The model under review builds one solid part; all positions refer to its coordinate system, in mm. A direction names the side the tool comes from. Round coordinates to 2 decimals unless told otherwise and drop trailing zeros. Order: outer loops, then holes, each group sorted by start corner. A loop starts at its lowest first (then second) coordinate and runs counter-clockwise, first axis right, second up. Notation, with made-up numbers: M 17.5,11.5 L 62.5,11.5 A29 cw 62.5,36.5 Z; hole C -33.75,-12.75 d8. An arc over 180 degrees is marked long. Use a Markdown table: item, result. Add a question column.
1. Insertion check: P1, Ø3, axis at y = -5, z = 5, coming from the -X side; P2, Ø6, axis at x = -8.5, z = 24, coming from the -Y side; P3, Ø1, axis at y = 7, z = 27, coming from the +X side; P4, Ø4, axis at x = 18.575, z = 22.5, coming from the -Y side. Each pin has a flat end and moves straight along its axis. Give the tip position at first contact, or say it passes through.
2. The part is to be moulded in two halves that separate along Z. For faces 3 (the flat face through (0, 6, 30)), 4 (the cylindrical face through (13.83, 1.2, 22.67)), 5 (the flat face through (-19, -8.55, 15)), say which applies: +Z half, -Z half, draft (parallel to the pull), parting line (faces both ways), or undercut.
3. To check wall thickness, follow probe 1 along Z at (x, y) = (-20.5, -7.75); probe 2 along X at (y, z) = (-6, 7.5) (3 decimals); probe 3 along X at (y, z) = (-4.5, 22.5) (3 decimals). State the ranges of each line that lie inside material, in increasing order.
4. Consider section C-C on y = 3. State the section outline as (x, z) points (3 decimals).
5. Consider section A-A on y = -3.75. State the section outline as (x, z) points (3 decimals), then the cut area to 3 significant figures.
6. For faces 1 (the flat face through (21, -2.25, 24)), 2 (the flat face through (-18.04, 2.71, 14.94)), list the 3-axis set-ups (+Z, -Z, +X, -X, +Y, -Y) from which the entire face can be reached by the end or side of a thin tool; tool diameter is ignored.
7. Consider section B-B on z = 22.5. State the section outline as (x, y) points (3 decimals).
from build123d import *

# Parameters (mm, degrees)
SKETCH1_W              = 48
SKETCH1_H              = 17.5
BODY_DEPTH             = 30
TUBE_CUTOUT_DEPTH      = 40.402569713
SKETCH3_R              = 2.65
CUT_EXTRUDE_M5_DEPTH   = 43.216702856
SLOPE_DEPTH            = 40.402569713
BOLT_HEAD_CUTOUT_START = -6.5
SKETCH5_R              = 4.75
BOLT_HEAD_CUTOUT_DEPTH = 23
FILLET_2_R             = 10
SKETCH7_W              = 48
SKETCH7_H              = 30
CLEARANCE_DEPTH        = 0.2


with BuildPart() as part:
    # Sketch1 → body (new body)
    with BuildSketch(Plane.XY):
        Rectangle(SKETCH1_W, SKETCH1_H)
    extrude(amount=BODY_DEPTH)

    # Sketch2 → tube_cutout (cut, through all)
    with BuildSketch(Plane.XY):
        with BuildLine():
            Line((13.15, -8.75), (-13.15, -8.75))
            ThreePointArc((-13.15, -8.75), (0, 4.4), (13.15, -8.75))
        make_face()
    extrude(amount=TUBE_CUTOUT_DEPTH, mode=Mode.SUBTRACT)

    # Sketch3 → Cut-Extrude M5 (cut, through all)
    with BuildSketch(Plane.XZ.offset(8.75)):
        with Locations(Location((18.575, 22.5, 0), (0, 0, 270))):
            Circle(SKETCH3_R)
        with Locations(Location((18.575, 7.5, 0), (0, 0, 270))):
            Circle(SKETCH3_R)
        with Locations(Location((-18.575, 7.5, 0), (0, 0, 90))):
            Circle(SKETCH3_R)
        with Locations(Location((-18.575, 22.5, 0), (0, 0, 90))):
            Circle(SKETCH3_R)
    extrude(amount=-CUT_EXTRUDE_M5_DEPTH, mode=Mode.SUBTRACT)

    # Sketch4 → slope (cut, through all)
    with BuildSketch(Plane.XY):
        Polygon((-24, 8.75), (-24, -3.25), (-12, 8.75), align=None)
        Polygon((24, -3.25), (12, 8.75), (24, 8.75), align=None)
    extrude(amount=SLOPE_DEPTH, mode=Mode.SUBTRACT)

    # Sketch5 → bolt_head_cutout (cut)
    with BuildSketch(Plane.XZ.offset(8.75).offset(BOLT_HEAD_CUTOUT_START)):
        with Locations((18.575, 22.5)):
            Circle(SKETCH5_R)
        with Locations((18.575, 7.5)):
            Circle(SKETCH5_R)
        with Locations((-18.575, 7.5)):
            Circle(SKETCH5_R)
        with Locations((-18.575, 22.5)):
            Circle(SKETCH5_R)
    extrude(amount=-BOLT_HEAD_CUTOUT_DEPTH, mode=Mode.SUBTRACT)

    # fillet 2
    # the kernel refuses this fillet: 10 mm, written as the material it takes off along each edge
    with BuildSketch(Plane(origin=(24, -3.25, -10.355339059), x_dir=(-0.7071067811865475, 0.7071067811865478, 0), z_dir=(0, 0, 1)), Plane(origin=(12, 8.75, -10.355339059), x_dir=(-1, 0, 0), z_dir=(0, 0, 1)), Plane(origin=(-12, 8.75, -10.355339059), x_dir=(-0.7071067811865474, -0.7071067811865478, 0), z_dir=(0, 0, 1))) as fillet_2_piece_1:
        with BuildLine():
            CenterArc((FILLET_2_R * 0.414213562373, FILLET_2_R), FILLET_2_R, 225, 45)
            Line((-FILLET_2_R * 0.292893218813, FILLET_2_R * 0.292893218813), (0, 0))
            Line((0, 0), (FILLET_2_R * 0.414213562373, 0))
        make_face()
    extrude(amount=50.710678119, mode=Mode.SUBTRACT)
    with BuildSketch(Plane(origin=(-24, -3.25, -10.355339059), x_dir=(0.7071067811865469, 0.707106781186548, 0), z_dir=(0, 0, 1))) as fillet_2_piece_2:
        with BuildLine():
            CenterArc((FILLET_2_R * 0.414213562373, -FILLET_2_R), FILLET_2_R, 90, 45)
            Line((-FILLET_2_R * 0.292893218813, -FILLET_2_R * 0.292893218813), (0, 0))
            Line((0, 0), (FILLET_2_R * 0.414213562373, 0))
        make_face()
    extrude(amount=50.710678119, mode=Mode.SUBTRACT)

    # Sketch7 → clearance (cut)
    with BuildSketch(Plane.XZ.offset(8.75)):
        with Locations((0, 15)):
            Rectangle(SKETCH7_W, SKETCH7_H)
    extrude(amount=-CLEARANCE_DEPTH, mode=Mode.SUBTRACT)


solid = part.part
Answer block:
| question | item | result |
|---|---|---|
| 1 | P1 | x = -23.96 |
| 1 | P2 | y = -2.37 |
| 1 | P3 | x = 14.18 |
| 1 | P4 | through |
| 2 | face 3 | +Z half |
| 2 | face 4 | undercut |
| 2 | face 5 | draft |
| 3 | probe 1 | 0 to 5.68, 9.32 to 20.68, 24.32 to 30 |
| 3 | probe 2 | -23.903 to -21.225, -15.925 to -12.859, 12.859 to 15.925, 21.225 to 23.903 |
| 3 | probe 3 | -23.573 to -21.225, -15.925 to -12.444, 12.444 to 15.925, 21.225 to 23.573 |
| 4 | outline | M -17.75,0 L -5.904,0 L -5.904,30 L -17.75,30 L -17.75,27.178 A4.75 cw -17.75,17.822 L -17.75,12.178 A4.75 cw -17.75,2.822 Z; M 5.904,0 L 17.75,0 L 17.75,2.822 A4.75 cw 17.75,12.178 L 17.75,17.822 A4.75 cw 17.75,27.178 L 17.75,30 L 5.904,30 Z |
| 5 | outline | M -23.313,0 L -12.162,0 L -12.162,30 L -23.313,30 Z; M 12.162,0 L 23.313,0 L 23.313,30 L 12.162,30 Z; hole C -18.575,7.5 d5.3; hole C -18.575,22.5 d5.3; hole C 18.575,7.5 d5.3; hole C 18.575,22.5 d5.3 |
| 5 | area | 581 mm^2 |
| 6 | face 1 | +Y |
| 6 | face 2 | +Z, -Z, -X, +Y |
| 7 | outline | M -24,-8.55 L -21.225,-8.55 L -21.225,-2.25 L -22.577,-2.25 A10 ccw -24,-7.392 Z; M -15.925,-8.55 L -13.148,-8.55 A13.15 cw 13.148,-8.55 L 15.925,-8.55 L 15.925,-2.25 L 13.825,-2.25 L 13.825,6.775 A10 ccw 7.858,8.75 L -7.858,8.75 A10 ccw -13.825,6.775 L -13.825,-2.25 L -15.925,-2.25 Z; M 21.225,-8.55 L 24,-8.55 L 24,-7.392 A10 ccw 22.577,-2.25 L 21.225,-2.25 Z |
